from build123d import *

# Parameters (mm, degrees)
SKETCH1_R           = 10
BOSS_EXTRUDE1_DEPTH = 10


with BuildPart() as part:
    # Sketch1 → Boss-Extrude1 (new body)
    with BuildSketch(Plane.XY):
        with BuildLine():
            Line((30.40998342, 7.530623632), (30.40998342, 16.840305532))
            Line((30.40998342, 16.840305532), (-26.463337265, 16.840305532))
            Line((-26.463337265, 16.840305532), (-26.463337265, -15.359839112))
            Line((-26.463337265, -15.359839112), (30.40998342, -15.359839112))
            Line((30.40998342, -15.359839112), (30.40998342, -2.10831855))
            Line((30.40998342, -2.10831855), (149.211555262, -2.10831855))
            ThreePointArc((149.211555262, -2.10831855), (198.71742784, 2.711152541), (149.211555262, 7.530623632))
            Line((149.211555262, 7.530623632), (30.40998342, 7.530623632))
        make_face()
        Circle(SKETCH1_R, mode=Mode.SUBTRACT)
    extrude(amount=BOSS_EXTRUDE1_DEPTH)


solid = part.part
Design review of the part built by this model. Coordinates are the model's own, in mm. A direction names the side the tool comes from. Coordinates: 2 decimals unless noted, no trailing zeros. Loops run counter-clockwise (first coordinate to the right, second up) from the corner with the lowest first, then second, coordinate; pieces in that order, holes last. Notation, with made-up numbers: (40.25, -4) - (53.25, -4) arc R16 cw to (53.25, 0) - close; hole circle Ø10 at (31, -18). An arc over 180 degrees is marked (long way). Use CSV: the item, a comma, the result in double quotes. Start each with the question number.
1. Add section C-C on z = 6.5. Give the boundary of the cut face in (x, y).
2. Add section D-D on x = 41. Give the boundary of the cut face in (y, z).
3. Clearance check with flat-ended pins moving along their axes: pin 1 (2 mm diameter, centred on x = 64, z = 8, fed in from -Y); pin 2 (1 mm diameter, centred on y = 11, z = 1.5, fed in from +X); pin 3 (2 mm diameter, centred on x = 25.5, z = 9, fed in from +Y). State where each tip first meets the part, or that it passes through.
4. For faces 1 (the flat face through (91, 7.531, 5)), 2 (the flat face through (110, 3, 0)), 3 (the flat face through (89, -2.108, 5)), 4 (the flat face through (2, 16.84, 5)), list the 3-axis set-ups (+Z, -Z, +X, -X, +Y, -Y) from which the entire face can be reached by the end or side of a thin tool; tool diameter is ignored.
5. Add section B-B on y = 0. Give the boundary of the cut face in (x, z).
6. Add section A-A on x = 0. Give the boundary of the cut face in (y, z).
7. Mouldability with a two-part tool opening along Y and no side actions: class faces 5 (the flat face through (2, -15.36, 5)), 6 (the cylindrical face through (-2.17, -9.76, 4.93)), 7 (the flat face through (-26.463, 1, 5)) as released by +Y, released by -Y, zero draft, split by the parting line, or undercut.
8. To check wall thickness, follow probe 1 along Y at (x, z) = (0, 6.25); probe 2 along Y at (x, z) = (63.5, 2.25); probe 3 along Y at (x, z) = (-11, 9.5). State the ranges of each line that lie inside material, in increasing order.
Resolved:
1,outline,"(-26.46, -15.36) - (30.41, -15.36) - (30.41, -2.11) - (149.21, -2.11) arc R24.99 ccw (long way) to (149.21, 7.53) - (30.41, 7.53) - (30.41, 16.84) - (-26.46, 16.84) - close; hole circle Ø20 at (0, 0)"
2,outline,"(-2.11, 0) - (7.53, 0) - (7.53, 10) - (-2.11, 10) - close"
3,pin 1,"y = -2.11"
3,pin 2,"x = 197.47"
3,pin 3,"y = 16.84"
4,face 1,"+Z, -Z, +Y"
4,face 2,"-Z, +X, -X, +Y, -Y"
4,face 3,"+Z, -Z, -Y"
4,face 4,"+Z, -Z, -X, +Y"
5,outline,"(-26.46, 0) - (-10, 0) - (-10, 10) - (-26.46, 10) - close; (10, 0) - (198.57, 0) - (198.57, 10) - (10, 10) - close"
6,outline,"(-15.36, 0) - (-10, 0) - (-10, 10) - (-15.36, 10) - close; (10, 0) - (16.84, 0) - (16.84, 10) - (10, 10) - close"
7,face 5,"released by -Y"
7,face 6,"undercut"
7,face 7,"zero draft"
8,probe 1,"-15.36 to -10, 10 to 16.84"
8,probe 2,"-2.11 to 7.53"
8,probe 3,"-15.36 to 16.84"
